Geometry: final body of the model. Coordinates: model frame, mm. A direction names the side the tool comes from. Round coordinates to 2 decimals unless told otherwise and drop trailing zeros. Loops run counter-clockwise (first coordinate to the right, second up) from the corner with the lowest first, then second, coordinate; pieces in that order, holes last. Notation, with made-up numbers: (50.25, 83) - (81.25, 83) arc R25 ccw to (81.25, 102) - close; hole circle Ø5 at (-33, -13.75). An arc over 180 degrees is marked (long way). Use CSV: the item, a comma, the result in double quotes.
from build123d import *

# Parameters (mm, degrees)
SKETCH1_W               = 100
SKETCH1_H               = 40
SKETCH1_R               = 7.6
BOSS_EXTRUDE4_DEPTH     = 5
SKETCH9_R               = 12.5
BOSS_EXTRUDE7_DEPTH     = 35
SKETCH1_7_W             = 100
SKETCH1_7_H             = 10
EXTRUDE_THIN1_DEPTH     = 40
BOSS_EXTRUDE5_DEPTH     = 5
BOSS_EXTRUDE6_DEPTH     = 5
SKETCH11_W              = 13
SKETCH11_H              = 11
CUT_EXTRUDE2_DEPTH      = 15
SKETCH13_5_R            = 3.25
CUT_EXTRUDE4_DEPTH      = 205
SKETCH13_R              = 3.25
CUT_EXTRUDE5_DEPTH      = 205
SKETCH15_W              = 29.641034448
SKETCH15_H              = 19.301138711
SKETCH15_W_2            = 23.765799192
SKETCH15_H_2            = 15.475404125
BOSS_EXTRUDE11_DEPTH    = 50
CUT_EXTRUDE6_DEPTH      = 32
CUT_EXTRUDE6_DEPTH_BACK = 66
SKETCH16_W              = 23.765799192
SKETCH16_H              = 15.475404125
SKETCH1_11_R            = 7.6
CUT_EXTRUDE1_DEPTH      = 25


with BuildPart() as part:
    # Sketch1 → Boss-Extrude4 (new body)
    with BuildSketch(Plane(origin=(0, 0, 0), x_dir=(1, 0, 0), z_dir=(0, 1, 0))):
        with Locations((0, -5)):
            Rectangle(SKETCH1_W, SKETCH1_H)
        with Locations(Location((0, 0, 0), (0, 0, 270))):
            Circle(SKETCH1_R, mode=Mode.SUBTRACT)
    extrude(amount=BOSS_EXTRUDE4_DEPTH)

    # Sketch9 → Boss-Extrude7 (add)
    with BuildSketch(Plane(origin=(0, 5, 0), x_dir=(1, 0, 0), z_dir=(0, 1, 0))):
        with Locations(Location((0, 0, 0), (0, 0, 270))):
            Circle(SKETCH9_R)
    extrude(amount=BOSS_EXTRUDE7_DEPTH)

    # Sketch1_7 → Extrude-Thin1 (add)
    with BuildSketch(Plane(origin=(0, 0, 0), x_dir=(1, 0, 0), z_dir=(0, 1, 0))):
        with Locations((0, 20)):
            Rectangle(SKETCH1_7_W, SKETCH1_7_H)
    extrude(amount=EXTRUDE_THIN1_DEPTH)

    # Sketch5 → Boss-Extrude5 (add)
    with BuildSketch(Plane(origin=(50, 0, 0), x_dir=(0, 0, -1), z_dir=(1, 0, 0))):
        Polygon((15, 40), (15, 5), (-25, 5), align=None)
    extrude(amount=-BOSS_EXTRUDE5_DEPTH)

    # Sketch6 → Boss-Extrude6 (add)
    with BuildSketch(Plane.ZY.offset(50)):
        Polygon((-15, 40), (-15, 5), (25, 5), align=None)
    extrude(amount=-BOSS_EXTRUDE6_DEPTH)

    # Sketch11 → Cut-Extrude2 (cut)
    with BuildSketch(Plane(origin=(0, 40, 0), x_dir=(1, 0, 0), z_dir=(0, 1, 0))):
        Rectangle(SKETCH11_W, SKETCH11_H)
    extrude(amount=-CUT_EXTRUDE2_DEPTH, mode=Mode.SUBTRACT)

    # Sketch13_5 → Cut-Extrude4 (cut)
    with BuildSketch(Plane(origin=(0, 0, -25), x_dir=(-1, 0, 0), z_dir=(0, 0, -1))):
        with Locations((30, 12.5)):
            Circle(SKETCH13_5_R)
    extrude(amount=-CUT_EXTRUDE4_DEPTH, mode=Mode.SUBTRACT)

    # Sketch13 → Cut-Extrude5 (cut)
    with BuildSketch(Plane(origin=(0, 0, -25), x_dir=(-1, 0, 0), z_dir=(0, 0, -1))):
        with Locations((-30, 12.5)):
            Circle(SKETCH13_R)
    extrude(amount=-CUT_EXTRUDE5_DEPTH, mode=Mode.SUBTRACT)

    # Sketch15 → Boss-Extrude11 (add)
    with BuildSketch(Plane(origin=(0, 0, -25), x_dir=(-1, 0, 0), z_dir=(0, 0, -1))):
        with Locations((0, 11.804714301)):
            Rectangle(SKETCH15_W, SKETCH15_H)
        with Locations((0, 11.804714301)):
            Rectangle(SKETCH15_W_2, SKETCH15_H_2, mode=Mode.SUBTRACT)
    extrude(amount=-BOSS_EXTRUDE11_DEPTH)

    # Sketch16 → Cut-Extrude6 (cut, two sides: drawn at the far end of the back side and taken through both)
    with BuildSketch(Plane(origin=(0, 0, -25), x_dir=(-1, 0, 0), z_dir=(0, 0, -1)).offset(-CUT_EXTRUDE6_DEPTH_BACK)):
        with Locations((0, 11.804714301)):
            Rectangle(SKETCH16_W, SKETCH16_H)
    extrude(amount=CUT_EXTRUDE6_DEPTH + CUT_EXTRUDE6_DEPTH_BACK, mode=Mode.SUBTRACT)

    # Sketch1_11 → Cut-Extrude1 (cut)
    with BuildSketch(Plane(origin=(0, 0, 0), x_dir=(1, 0, 0), z_dir=(0, 1, 0))):
        with Locations(Location((0, 0, 0), (0, 0, 90))):
            Circle(SKETCH1_11_R)
    extrude(amount=CUT_EXTRUDE1_DEPTH, mode=Mode.SUBTRACT)


solid = part.part
Item 1: Section D-D on z = -18.5. Return the cut outline in (x, y).
Final values:
outline,"(-50, 0) - (50, 0) - (50, 40) - (-50, 40) - close; hole circle Ø6.5 at (-30, 12.5); hole (-11.88, 4.07) - (11.88, 4.07) - (11.88, 19.54) - (-11.88, 19.54) - close; hole circle Ø6.5 at (30, 12.5)"
Item 2: Mould query, pull axis Z, two halves, no side actions, for faces 1 (the flat face through (47.535, 22.255, 5.28)), 2 (the flat face through (0, 21.455, 14)), 3 (the flat face through (0, 40, -6)). Classes: released by +Z, released by -Z, zero draft, split by the parting line, or undercut.
Final values:
face 1,"released by +Z"
face 2,"undercut"
face 3,"zero draft"
Item 3: Section A-A on x = 30. Return the cut outline in (y, z), plus the area to 3 significant figures.
Final values:
outline,"(0, -25) - (9.25, -25) - (9.25, -15) - (5, -15) - (5, 25) - (0, 25) - close; (15.75, -25) - (40, -25) - (40, -15) - (15.75, -15) - close"
area,"535 mm²"
Item 4: Reachability of faces 4 (the cylindrical face through (7.583, 2.005, 0.501)), 5 (the flat face through (-30, 5, 5)), 6 (the flat face through (-6.5, 33, 0)) from +Z, -Z, +X, -X, +Y, -Y: full face, straight path, thin tool, end or side. Return the list, or none.
Final values:
face 4,"-Y"
face 5,"+Z, +Y"
face 6,"+Y"
Item 5: Section B-B on y = 27. Return the cut outline in (x, z), plus the area to 3 significant figures.
Final values:
outline,"(-50, -25) - (50, -25) - (50, -0.14) - (45, -0.14) - (45, -15) - (-45, -15) - (-45, -0.14) - (-50, -0.14) - close; circle Ø25 at (0, 0); hole (-6.5, -5.5) - (6.5, -5.5) - (6.5, 5.5) - (-6.5, 5.5) - close"
area,"1,500 mm²"
Item 6: Pin query (flat end, axial travel): P1, Ø14.5, axis at x = 1.5, y = 31.5, coming from the +Z side; P2, Ø1, axis at x = 35.5, y = 9.5, coming from the +Z side; P3, Ø13.5, axis at x = 0, z = 0, coming from the -Y side; P4, Ø9, axis at x = 0, z = 0, coming from the -Y side. Return the tip coordinate at first contact, or that it passes through.
Final values:
P1,"stops at z = 12.5"
P2,"stops at z = -15"
P3,"stops at y = 25"
P4,"passes through"
Item 7: Material intervals for line 1 (X direction, y = 12.5, z = 14); line 2 (Y direction, x = 8.5, z = 22); line 3 (X direction, y = 9, z = 21.5), sorted ascending.
Final values:
line 1,"x = -50 to -45, -14.82 to -11.88, 11.88 to 14.82, 45 to 50"
line 2,"y = 0 to 4.07, 19.54 to 21.46"
line 3,"x = -14.82 to -11.88, 11.88 to 14.82"
